Source: CAD feature listing. Evaluate the final solid. Frame: model axes, mm. Give positions to 0.01 mm unless a question says otherwise; leave off trailing zeros. Order: outer loops, then holes, each group sorted by start corner. A loop starts at its lowest first (then second) coordinate and runs counter-clockwise, first axis right, second up. Notation, with made-up numbers: (-37.75, 12.5) - (3.25, 12.5) arc R7 ccw to (3.25, 19.5) - close; hole circle Ø9 at (-10, 74.25). An arc over 180 degrees is marked (long way). Use CSV: the item, a comma, the result in double quotes.
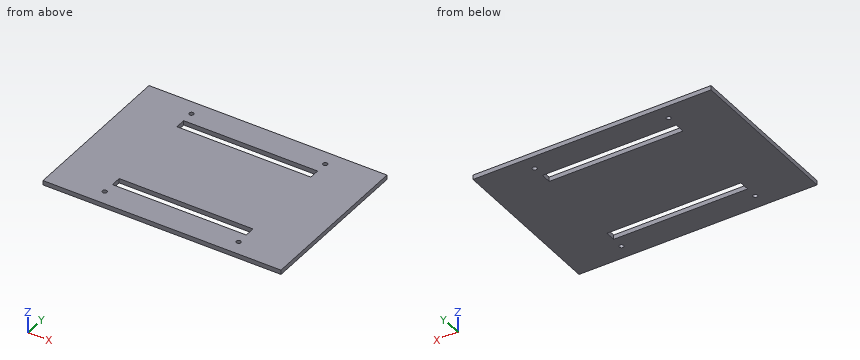
```python
from build123d import *

# Parameters (mm, degrees)
SKETCH1_W           = 160
SKETCH1_H           = 110
SKETCH1_R           = 1.5
SKETCH1_W_2         = 90
SKETCH1_H_2         = 7
BOSS_EXTRUDE1_DEPTH = 3


with BuildPart() as part:
    # Sketch1 → Boss-Extrude1 (new body)
    with BuildSketch(Plane.XY):
        Rectangle(SKETCH1_W, SKETCH1_H)
        with Locations((45, 45)):
            Circle(SKETCH1_R, mode=Mode.SUBTRACT)
        with Locations((-45, 45)):
            Circle(SKETCH1_R, mode=Mode.SUBTRACT)
        with Locations((-45, -45)):
            Circle(SKETCH1_R, mode=Mode.SUBTRACT)
        with Locations((45, -45)):
            Circle(SKETCH1_R, mode=Mode.SUBTRACT)
        with Locations((0, 33.5)):
            Rectangle(SKETCH1_W_2, SKETCH1_H_2, mode=Mode.SUBTRACT)
        with Locations((0, -33.5)):
            Rectangle(SKETCH1_W_2, SKETCH1_H_2, mode=Mode.SUBTRACT)
    extrude(amount=BOSS_EXTRUDE1_DEPTH)


solid = part.part
```
Item 1: First-contact query: pin 1 (3 mm diameter, centred on x = 41, y = -43, fed in from -Z). Flat tip, straight axial feed; report the tip coordinate or a pass-through.
Filled in:
pin 1,"stops at z = 0"
Item 2: Material intervals for line 1 (X direction, y = 32, z = 2.8); line 2 (Y direction, x = 16, z = 2.3), sorted ascending. Write a range as from..to.
Filled in:
line 1,"x = -80..-45, 45..80"
line 2,"y = -55..-37, -30..30, 37..55"
Item 3: Section B-B on x = -1. Return the cut outline in (y, z).
Filled in:
outline,"(-55, 0) - (-37, 0) - (-37, 3) - (-55, 3) - close; (-30, 0) - (30, 0) - (30, 3) - (-30, 3) - close; (37, 0) - (55, 0) - (55, 3) - (37, 3) - close"
Item 4: Section A-A on z = 0.75. Return the cut outline in (x, y).
Filled in:
outline,"(-80, -55) - (80, -55) - (80, 55) - (-80, 55) - close; hole circle Ø3 at (-45, -45); hole circle Ø3 at (-45, 45); hole (-45, -37) - (45, -37) - (45, -30) - (-45, -30) - close; hole (-45, 30) - (45, 30) - (45, 37) - (-45, 37) - close; hole circle Ø3 at (45, -45); hole circle Ø3 at (45, 45)"
